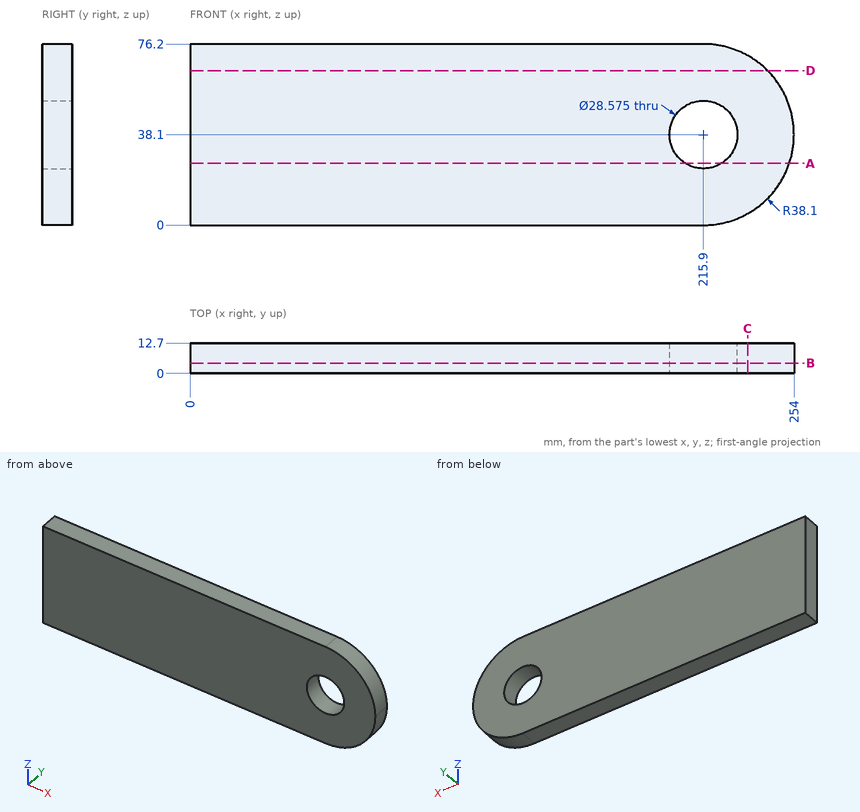
Input: dimensioned drawing with shaded views. Units: mm. Origin: part minimum x, y, z. Give positions to 0.01 mm unless a question says otherwise; leave off trailing zeros. Write each loop counter-clockwise with the first axis right and the second up, starting at its lowest first coordinate (ties: lowest second). Pieces come first, ordered by that corner, then holes. Notation, with made-up numbers: (21, -11.75) - (37, -11.75) arc R13 ccw to (37, -4.75) - close; hole circle Ø7 at (89.25, 28.5). An arc over 180 degrees is marked (long way). One line per item, written item: value. Start each with the question number.
Q1. Section query B-B, the plane y = 4.25. Return the cut outline in (x, z) (1 decimal), then the cut area to 3 significant figures.
Q2. Section query D-D, the plane z = 65. Return the cut outline in (x, y).
Q3. First-contact query: pin 1 Ø23 at (x, z) = (215.9, 38.1) entering from -Y. Flat tip, straight axial feed; report the tip coordinate or a pass-through.
Q4. Section query C-C, the plane x = 234.5. Return the cut outline in (y, z), then the cut area to 3 significant figures.
Q5. Material intervals for probe 1 along Z at (x, y) = (215.9, 8.75); probe 2 along X at (y, z) = (1.25, 38); probe 3 along X at (y, z) = (9.25, 27), sorted ascending. Write a range as from..to.
Q6. Section query A-A, the plane z = 26. Return the cut outline in (x, y).
Answer:
1. outline: (0, 0) - (215.9, 0) arc R38.1 ccw to (254, 38.1) arc R38.1 ccw to (215.9, 76.2) - (0, 76.2) - close; hole circle Ø28.6 at (215.9, 38.1)
1. area: 18,100 mm2
2. outline: (0, 0) - (242.88, 0) - (242.88, 12.7) - (0, 12.7) - close
3. pin 1: passes through
4. outline: (0, 4.85) - (12.7, 4.85) - (12.7, 71.35) - (0, 71.35) - close
4. area: 845 mm2
5. probe 1: z = 0..23.81, 52.39..76.2
5. probe 2: x = 0..201.61, 230.19..254
5. probe 3: x = 0..206.9, 224.9..252.35
6. outline: (0, 0) - (208.3, 0) - (208.3, 12.7) - (0, 12.7) - close; (223.5, 0) - (252.03, 0) - (252.03, 12.7) - (223.5, 12.7) - close
